Verification items for the finished model (mm, model axes). A direction names the side the tool comes from. Give positions to 0.01 mm unless a question says otherwise; leave off trailing zeros. Loops run counter-clockwise (first coordinate to the right, second up) from the corner with the lowest first, then second, coordinate; pieces in that order, holes last. Notation, with made-up numbers: M -13,72.5 L 31,72.5 A20 ccw 31,78.5 Z; hole C 72.25,-12.5 d6. An arc over 180 degrees is marked long. Use a Markdown table: item, result.
from build123d import *

# Parameters (mm, degrees)
F0_R     = 6
F0_W     = 20
F0_H     = 40
F1_DEPTH = 60


with BuildPart() as f1:
    # F0 (on Top) → F1 (new body)
    with BuildSketch(Plane.XY):
        with BuildLine():
            Line((-48.008848, 52.76), (-53.205, 49.76))
            Line((-53.205, 49.76), (-16.535, -13.754303))
            Line((-16.535, -13.754303), (-33.855508, -23.754303))
            Line((-33.855508, -23.754303), (-21.727863, -44.76))
            ThreePointArc((-21.727863, -44.76), (-18.067609, -48.420254), (-13.067609, -49.76))
            Line((-13.067609, -49.76), (13.067609, -49.76))
            ThreePointArc((13.067609, -49.76), (18.067609, -48.420254), (21.727863, -44.76))
            Line((21.727863, -44.76), (33.855508, -23.754303))
            Line((33.855508, -23.754303), (16.535, -13.754303))
            Line((16.535, -13.754303), (53.205, 49.76))
            Line((53.205, 49.76), (48.008848, 52.76))
            Line((48.008848, 52.76), (40.636085, 39.99))
            ThreePointArc((40.636085, 39.99), (37.707881, 37.061797), (33.707881, 35.99))
            Line((33.707881, 35.99), (-33.707881, 35.99))
            ThreePointArc((-33.707881, 35.99), (-37.707881, 37.061797), (-40.636085, 39.99))
            Line((-40.636085, 39.99), (-48.008848, 52.76))
        make_face()
        with Locations((-20.445254, -26.981544)):
            Circle(F0_R, mode=Mode.SUBTRACT)
        with Locations((20.445254, -26.981544)):
            Circle(F0_R, mode=Mode.SUBTRACT)
        with Locations((0, -23.76)):
            Rectangle(F0_W, F0_H, mode=Mode.SUBTRACT)
        with BuildLine():
            ThreePointArc((22.882564, 9.24), (19.22231, 5.579746), (14.22231, 4.24))
            Line((14.22231, 4.24), (-14.22231, 4.24))
            ThreePointArc((-14.22231, 4.24), (-19.22231, 5.579746), (-22.882564, 9.24))
            Line((-22.882564, 9.24), (-34.285232, 28.99))
            ThreePointArc((-34.285232, 28.99), (-34.285232, 30.99), (-32.553181, 31.99))
            Line((-32.553181, 31.99), (32.553181, 31.99))
            ThreePointArc((32.553181, 31.99), (34.285232, 30.99), (34.285232, 28.99))
            Line((34.285232, 28.99), (22.882564, 9.24))
        make_face(mode=Mode.SUBTRACT)
    extrude(amount=F1_DEPTH)


solid = f1.part
(1) Cross-section at B-B on y = 37.5. Record the cut outline in (x, z), then the cut area to 3 significant figures.
Results below:
| item | result |
|---|---|
| outline | M -46.13,0 L -38.39,0 L -38.39,60 L -46.13,60 Z; M 38.39,0 L 46.13,0 L 46.13,60 L 38.39,60 Z |
| area | 929 mm^2 |
(2) Gauge pin test, flat ends, axial feed: P1, Ø10, axis at y = -32.5, z = 29, coming from the -X side; P2, Ø10, axis at x = -1.5, z = 24.5, coming from the +Y side; P3, Ø6, axis at x = -34.5, z = 24, coming from the -Y side. Record the tip position at first contact, or that the pin passes through.
Results below:
| item | result |
|---|---|
| P1 | x = -31.69 |
| P2 | y = 35.99 |
| P3 | y = -27.83 |
(3) Draft check along X on faces 1 (the cylindrical face through (-18.1, -48.4, 29.6)), 2 (the flat face through (-4, 2, 60)), 3 (the flat face through (-44.271, 46.286, 29.58)). Enter one of: +X half, -X half, draft (parallel to the pull), parting line (faces both ways), or undercut.
Results below:
| item | result |
|---|---|
| face 1 | -X half |
| face 2 | draft |
| face 3 | undercut |
(4) Cross-section at A-A on x = -0.5. Record the cut outline in (y, z), then the cut area to 3 significant figures.
Results below:
| item | result |
|---|---|
| outline | M -49.76,0 L -43.76,0 L -43.76,60 L -49.76,60 Z; M -3.76,0 L 4.24,0 L 4.24,60 L -3.76,60 Z; M 31.99,0 L 35.99,0 L 35.99,60 L 31.99,60 Z |
| area | 1,080 mm^2 |
(5) Set-up check for faces 4 (the flat face through (-35.1, 18.4, 29.6)), 5 (the cylindrical face through (-34.3, 30.96, 29.58)), 6 (the flat face through (25.316, -18.824, 29.58)), 7 (the cylindrical face through (-37.657, 37.033, 29.58)): record each of +Z, -Z, +X, -X, +Y, -Y from which the full face is reachable in a straight line by a thin tool's end or side.
Results below:
| item | result |
|---|---|
| face 4 | +Z, -Z, -X |
| face 5 | +Z, -Z |
| face 6 | +Z, -Z, +X |
| face 7 | +Z, -Z, +Y |
(6) Cross-section at D-D on x = -38.5. Record the cut outline in (y, z), then the cut area to 3 significant figures.
Results below:
| item | result |
|---|---|
| outline | M 24.29,0 L 37.58,0 L 37.58,60 L 24.29,60 Z |
| area | 798 mm^2 |
(7) Cross-section at C-C on z = 4. State how many separate pieces and enclosed holes the cut face has, then the cut area to 3 significant figures.
Results below:
| item | result |
|---|---|
| separate pieces | 1 |
| enclosed holes | 4 |
| area | 2,590 mm^2 |
(8) Material ranges on line 1 (Y direction, x = 9, z = 41); line 2 (Y direction, x = 26.5, z = 14); line 3 (Y direction, x = -21, z = 14.5), recorded low to high.
Results below:
| item | result |
|---|---|
| line 1 | -49.76 to -43.76, -3.76 to 4.24, 31.99 to 35.99 |
| line 2 | -36.49 to -19.51, 3.51 to 15.51, 31.99 to 35.99 |
| line 3 | -45.85 to -32.96, -21.01 to -16.33, -6.02 to 6.89, 31.99 to 35.99 |
